Can you work these out from the model? Positions are in its coordinate system, mm. A direction names the side the tool comes from. Coordinates: 2 decimals unless noted, no trailing zeros. Loops run counter-clockwise (first coordinate to the right, second up) from the corner with the lowest first, then second, coordinate; pieces in that order, holes last.
```python
from build123d import *

# Parameters (mm, degrees)
SKETCH1_R           = 2.5
BOSS_EXTRUDE1_DEPTH = 6
CUT_EXTRUDE2_DEPTH  = 3


with BuildPart() as part:
    # Sketch1 → Boss-Extrude1 (new body)
    with BuildSketch(Plane.XY):
        with BuildLine():
            Line((30, 5), (0, 5))
            ThreePointArc((0, 5), (-3.535533906, 3.535533906), (-5, 0))
            Line((-5, 0), (-5, -43.530327794))
            ThreePointArc((-5, -43.530327794), (-1.289471128, -48.361193576), (4.334905684, -46.022032574))
            Line((4.334905684, -46.022032574), (19.026166695, -20.463133553))
            Line((19.026166695, -20.463133553), (19.026166695, -5))
            Line((19.026166695, -5), (30, -5))
            ThreePointArc((30, -5), (35, 0), (30, 5))
        make_face()
        Circle(SKETCH1_R, mode=Mode.SUBTRACT)
        with Locations((30, 0)):
            Circle(SKETCH1_R, mode=Mode.SUBTRACT)
    extrude(amount=-BOSS_EXTRUDE1_DEPTH)

    # Sketch3 → Cut-Extrude2 (cut)
    with BuildSketch(Plane.XY):
        with BuildLine():
            Line((12.275244192, 5), (12.275244192, -7.004190344))
            Line((12.275244192, -7.004190344), (-5, -7.004190344))
            Line((-5, -7.004190344), (-5, 0))
            ThreePointArc((-5, 0), (-3.535533906, 3.535533906), (0, 5))
            Line((0, 5), (12.275244192, 5))
        make_face()
    extrude(amount=-CUT_EXTRUDE2_DEPTH, mode=Mode.SUBTRACT)


solid = part.part
```
(1) If we mould it in two halves opening along Y, with no side actions, what happens to faces 4 (the flat face through (24, -5, -3)), 5 (the flat face through (-5, -21, -3)), 6 (the cylindrical face through (-0.54, -2.44, -4.48))? For each: released by +Y, released by -Y, zero draft, split by the parting line, or undercut.
Check values:
face 4: released by -Y
face 5: zero draft
face 6: undercut
(2) Which directions (+Z, -Z, +X, -X, +Y, -Y) give clear straight access to the entire face, cutting with the end or side of a thin tool? Please do faces 1 (the flat face through (19.026, -13, -3)), 2 (the flat face through (12.275, -1, -1)), 3 (the flat face through (10, -15, 0)).
Check values:
face 1: +Z, -Z, +X, -Y
face 2: +Z, -X, +Y
face 3: +Z, +X, -X, +Y, -Y
(3) If I drill on probe 1 along Y at (x, z) = (0, -4.45); probe 2 along Y at (x, z) = (22.5, -1.25); probe 3 along Y at (x, z) = (30, -2.6), over which ranges is the centre line in solid material (lowest first)?
Check values:
probe 1: y = -48.53 to -2.5, 2.5 to 5
probe 2: y = -5 to 5
probe 3: y = -5 to -2.5, 2.5 to 5
(4) I want a section at B-B on x = 31. Write out the boundary of the cut face in (y, z).
Check values:
outline: (-4.9, -6) - (-2.29, -6) - (-2.29, 0) - (-4.9, 0) - close; (2.29, -6) - (4.9, -6) - (4.9, 0) - (2.29, 0) - close
(5) I want a section at D-D on x = 11. Write out the boundary of the cut face in (y, z), then the cut area to 3 significant figures.
Check values:
outline: (-34.43, -6) - (5, -6) - (5, -3) - (-7, -3) - (-7, 0) - (-34.43, 0) - close
area: 201 mm2
(6) I'm going to push flat-ended pins straight in: pin 1 (1.5 mm diameter, centred on x = 3, z = -1.5, fed in from +Y); pin 2 (3.5 mm diameter, centred on x = 1.5, y = 0.5, fed in from +Z); pin 3 (1.8 mm diameter, centred on x = 24.5, z = -4, fed in from -Y). Where does each tip first touch, or does it pass through?
Check values:
pin 1: stops at y = -7
pin 2: stops at z = -3
pin 3: stops at y = -5
(7) I want a section at C-C on y = -10.5. Write out the boundary of the cut face in (x, z), then the cut area to 3 significant figures.
Check values:
outline: (-5, -6) - (19.03, -6) - (19.03, 0) - (-5, 0) - close
area: 144 mm2
(8) I want a section at A-A on z = -5.45. Write out the boundary of the cut face in (x, y).
Check values:
outline: (-5, -43.53) arc R5 ccw to (4.33, -46.02) - (19.03, -20.46) - (19.03, -5) - (30, -5) arc R5 ccw to (30, 5) - (0, 5) arc R5 ccw to (-5, 0) - close; hole circle Ø5 at (0, 0); hole circle Ø5 at (30, 0)
